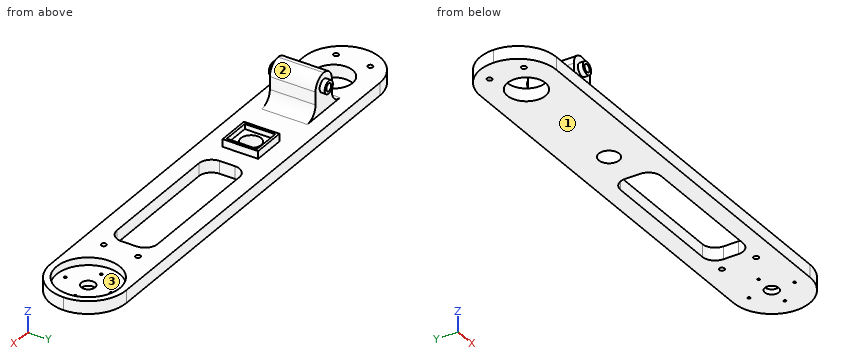
```python
from build123d import *
from build123d import SkipClean  # not in build123d's __all__

# Parameters (mm, degrees)
F0_W      = 185
F0_H      = 30
F0_R      = 1
F0_W_2    = 60
F0_H_2    = 16
F1_DEPTH  = 5
F2_R      = 12.5
F2_R_2    = 0.5
F2_R_3    = 2.75
F3_DEPTH  = 3
F4_DEPTH  = 25
F5_R      = 14.99999
F2_R_4    = 7.5
F6_DEPTH  = 25
F2_W      = 10
F2_H      = 18
F7_DEPTH  = 15
F8_R      = 4.99999
F9_R      = 1.5
F10_DEPTH = 25
F9_R_2    = 2.5
F11_DEPTH = 2
F12_R     = 2.5
F12_R_2   = 1.5
F13_DEPTH = 2
F2_W_2    = 13
F2_H_2    = 14
F14_DEPTH = 3
F15_W     = 11
F15_H     = 12
F15_R     = 4
F16_DEPTH = 2
F17_DEPTH = 25
F18_R     = 5


# Not quite as in the source:
# - a fillet or chamfer is up to 0.001 mm smaller than in the source, because OpenCascade refuses the exact size
# - after a boolean that leaves OpenCascade's solid faulty, fix() repairs it


with BuildPart() as f1:
    # F0 (on Top) → F1 (new body)
    with BuildSketch(Plane.XY):
        with Locations((7.5, -11.8972941886)):
            Rectangle(F0_W, F0_H)
        with Locations((-77, -18.6472941886)):
            Circle(F0_R, mode=Mode.SUBTRACT)
        with Locations((30, -11.8972941886)):
            Rectangle(F0_W_2, F0_H_2, mode=Mode.SUBTRACT)
        with Locations((65, -18.6472941886)):
            Circle(F0_R, mode=Mode.SUBTRACT)
        with Locations((-77, -5.1472941886)):
            Circle(F0_R, mode=Mode.SUBTRACT)
        with Locations((65, -5.1472941886)):
            Circle(F0_R, mode=Mode.SUBTRACT)
    extrude(amount=F1_DEPTH)

    # F2 (on face) → F3 (cut)
    with BuildSketch(Plane.XY.offset(5)):
        with Locations((85, -11.8972941886)):
            Circle(F2_R)
        with Locations((85, -20.8972941886)):
            Circle(F2_R_2, mode=Mode.SUBTRACT)
        with Locations((85, -11.8972941886)):
            Circle(F2_R_3, mode=Mode.SUBTRACT)
        with Locations((77, -11.8972941886)):
            Circle(F2_R_2, mode=Mode.SUBTRACT)
        with Locations((93, -11.8972941886)):
            Circle(F2_R_2, mode=Mode.SUBTRACT)
        with Locations((85, -2.8972941886)):
            Circle(F2_R_2, mode=Mode.SUBTRACT)
    extrude(amount=-F3_DEPTH, mode=Mode.SUBTRACT)

    # F2 (on face) → F4 (cut)
    with BuildSketch(Plane.XY.offset(5)):
        with Locations((85, -11.8972941886)):
            Circle(F2_R_3)
        with Locations((85, -2.8972941886)):
            Circle(F2_R_2)
        with Locations((77, -11.8972941886)):
            Circle(F2_R_2)
        with Locations((85, -20.8972941886)):
            Circle(F2_R_2)
        with Locations((93, -11.8972941886)):
            Circle(F2_R_2)
    extrude(amount=-F4_DEPTH, mode=Mode.SUBTRACT)

    # F5 (radius 15 in the source; OpenCascade refuses exactly that, so slightly less here)
    f5_edges = [f1.edges().sort_by_distance(p)[0] for p in [
        (100, 3.102706, 2.5),
        (100, -26.897294, 2.5),
        (-85, -26.897294, 2.5),
        (-85, 3.102706, 2.5),
    ]]
    fillet(f5_edges, radius=F5_R)

    # F2 (on face) → F6 (cut)
    with BuildSketch(Plane.XY.offset(5)):
        with Locations((-65, -11.8972941886)):
            Circle(F2_R_4)
    extrude(amount=-F6_DEPTH, mode=Mode.SUBTRACT)

    # F2 (on face) → F7 (join)
    with BuildSketch(Plane.XY.offset(5)):
        with Locations((-45, -11.8972941886)):
            Rectangle(F2_W, F2_H)
    extrude(amount=F7_DEPTH)

    # F8 (radius 5 in the source; OpenCascade refuses exactly that, so slightly less here)
    f8_edges = [f1.edges().sort_by_distance(p)[0] for p in [
        (-50, -11.897294, 5),
        (-40, -11.897294, 20),
        (-50, -11.897294, 20),
        (-40, -11.897294, 5),
    ]]
    fillet(f8_edges, radius=F8_R)

    # F9 (on face) → F10 (cut)
    with BuildSketch(Plane.XZ.offset(20.8972941886)):
        with Locations((-45, 15)):
            Circle(F9_R)
    extrude(amount=-F10_DEPTH, mode=Mode.SUBTRACT)

    # F9 (on face) → F11 (join)
    with BuildSketch(Plane.XZ.offset(20.8972941886)):
        with Locations((-45, 15)):
            Circle(F9_R_2)
        with Locations((-45, 15)):
            Circle(F9_R, mode=Mode.SUBTRACT)
    extrude(amount=F11_DEPTH)

    # F12 (on face) → F13 (join)
    with BuildSketch(Plane(origin=(0, -2.8972941886, 0), x_dir=(-1, 0, 0), z_dir=(0, 1, 0))):
        with Locations((45, 15)):
            Circle(F12_R)
        with Locations((45, 15)):
            Circle(F12_R_2, mode=Mode.SUBTRACT)
    with SkipClean():  # cleaning this boolean's faces spoils the solid; the shape is the same uncleaned
        extrude(amount=F13_DEPTH)

    # F2 (on face) → F14 (join)
    with BuildSketch(Plane.XY.offset(5)):
        with Locations((-14.5, -11.8972941886)):
            Rectangle(F2_W_2, F2_H_2)
    extrude(amount=F14_DEPTH)

    add(f1.part.fix(), mode=Mode.REPLACE)

    # F15 (on face) → F16 (cut)
    with BuildSketch(Plane.XY.offset(8)):
        with Locations((-14.5, -11.8972941886)):
            Rectangle(F15_W, F15_H)
        with Locations((-14.5, -11.8972941886)):
            Circle(F15_R, mode=Mode.SUBTRACT)
    extrude(amount=-F16_DEPTH, mode=Mode.SUBTRACT)

    # F17 (cut): a face of the model
    f17_faces = [f1.faces().sort_by_distance(p)[0] for p in [
        (-14.5, -11.8972941886, 8),
    ]]
    extrude(f17_faces, amount=-F17_DEPTH, mode=Mode.SUBTRACT)

    # F18
    f18_edges = [f1.edges().sort_by_distance(p)[0] for p in [
        (0, -3.897294, 2.5),
        (0, -19.897294, 2.5),
        (60, -3.897294, 2.5),
        (60, -19.897294, 2.5),
    ]]
    fillet(f18_edges, radius=F18_R)


solid = f1.part
```
CAD build for the part. Positions are in the model's coordinates, mm. Face numbers are marked on the shaded views. Give positions to 0.01 mm unless a question says otherwise; leave off trailing zeros. Order: outer loops, then holes, each group sorted by start corner. A loop starts at its lowest first (then second) coordinate and runs counter-clockwise, first axis right, second up. Notation, with made-up numbers: M 45.5,5.5 L 68.5,5.5 A16 ccw 68.5,29.5 Z; hole C 34,-33 d4. An arc over 180 degrees is marked long. Put each result on its own line as item: value. Start each with the question number.
(1) Saw through at C-C, the plane x = -13. Write the cut outline in (y, z).
(2) Mould opens along X. For the marked faces 1, 2 and 3 say: +X half, -X half, draft (parallel to the pull), parting line (faces both ways), or undercut.
(3) Flat gauge pins, fed straight in: pin 1 Ø4 at (x, y) = (22.5, -21) entering from +Z; pin 2 Ø2.5 at (x, z) = (-44.5, 14) entering from -Y; pin 3 Ø1.6 at (x, z) = (-12.5, 7.5) entering from -Y. Where does each tip first touch, or does it go through?
(4) Saw through at B-B, the plane x = 26.5. Write the cut outline in (y, z), then the cut area to 3 significant figures.
(5) Saw through at A-A, the plane x = -65. Write the cut outline in (y, z).
(6) Drill centre lines: line 1 along Z through (x, y) = (-45, -21.65); line 2 along Y through (x, z) = (65, 3.3); line 3 along X through (y, z) = (-13.5, 2.5). Where is each one in solid material? Low to high.
Check result:
1. outline: M -26.9,0 L -15.61,0 L -15.61,6 L -17.9,6 L -17.9,8 L -18.9,8 L -18.9,5 L -26.9,5 Z; M -8.19,0 L 3.1,0 L 3.1,5 L -4.9,5 L -4.9,8 L -5.9,8 L -5.9,6 L -8.19,6 Z
2. face 1: draft
2. face 2: +X half
2. face 3: undercut
3. pin 1: stops at z = 5
3. pin 2: stops at y = -22.9
3. pin 3: stops at y = -18.9
4. outline: M -26.9,0 L -19.9,0 L -19.9,5 L -26.9,5 Z; M -3.9,0 L 3.1,0 L 3.1,5 L -3.9,5 Z
4. area: 70.0 mm2
5. outline: M -26.9,0 L -19.4,0 L -19.4,5 L -26.9,5 Z; M -4.4,0 L 3.1,0 L 3.1,5 L -4.4,5 Z
6. line 1: z = 0 to 5, 12.5 to 13.5, 16.5 to 17.5
6. line 2: y = -26.9 to -19.65, -17.65 to -6.15, -4.15 to 3.1
6. line 3: x = -84.91 to -72.33, -57.67 to -18.16, -10.84 to 0, 60 to 72.6, 97.4 to 99.91
